from build123d import *

# Parameters (mm, degrees)
BOSS_EXTRUDE1_DEPTH = 3


with BuildPart() as part:
    # Sketch1 → Boss-Extrude1 (new body)
    with BuildSketch(Plane.XY):
        with BuildLine():
            Line((-5, -4), (-5, 4))
            ThreePointArc((-5, 4), (0, 9), (5, 4))
            Line((5, 4), (5, -4))
            ThreePointArc((5, -4), (0, -9), (-5, -4))
        make_face()
        Polygon((1.616580754, 1.2), (3.233161507, 4), (1.616580754, 6.8), (-1.616580754, 6.8), (-3.233161507, 4), (-1.616580754, 1.2), align=None, mode=Mode.SUBTRACT)
        Polygon((3.233161507, -4), (1.616580754, -1.2), (-1.616580754, -1.2), (-3.233161507, -4), (-1.616580754, -6.8), (1.616580754, -6.8), align=None, mode=Mode.SUBTRACT)
    extrude(amount=BOSS_EXTRUDE1_DEPTH)


solid = part.part
Design review of the part built by this model. Coordinates are the model's own, in mm. A direction names the side the tool comes from. Round coordinates to 2 decimals unless told otherwise and drop trailing zeros. Write each loop counter-clockwise with the first axis right and the second up, starting at its lowest first coordinate (ties: lowest second). Pieces come first, ordered by that corner, then holes. Notation, with made-up numbers: (39, 80.25) -> (62, 80.25) arc R25 ccw to (62, 113.25) -> close; hole circle Ø5 at (-30, 20). An arc over 180 degrees is marked (long way). One line per question, with ' | ' between items.
(1) Take a section at C-C, the plane y = 2.75. State the section outline as (x, z) points.
Result sheet:
outline: (-5, 0) -> (-2.51, 0) -> (-2.51, 3) -> (-5, 3) -> close; (2.51, 0) -> (5, 0) -> (5, 3) -> (2.51, 3) -> close
(2) Take a section at D-D, the plane y = -7. State the section outline as (x, z) points, and give its area (3 significant figures).
Result sheet:
outline: (-4, 0) -> (4, 0) -> (4, 3) -> (-4, 3) -> close | area: 24.0 mm2
(3) Wall thickness on line 1 (Y direction, x = 2.25, z = 0.6); line 2 (Y direction, x = 0, z = 1); line 3 (X direction, y = -5.5, z = 1.15): over which ranges is each line inside the solid? List them lowest first. Write a range as [from, to].
Result sheet:
line 1: [-8.47, -5.7], [-2.3, 2.3], [5.7, 8.47] | line 2: [-9, -6.8], [-1.2, 1.2], [6.8, 9] | line 3: [-4.77, -2.37], [2.37, 4.77]
(4) Draft analysis for pull direction Y (two halves, no side actions). For faces 3 (the flat face through (-2.436, 2.62, 1.479)), 4 (the cylindrical face through (0, -9, 1)), 5 (the flat face through (-5, 0, 1)), state which applies: released by +Y, released by -Y, zero draft, split by the parting line, or undercut.
Result sheet:
face 3: undercut | face 4: released by -Y | face 5: zero draft
(5) Take a section at B-B, the plane z = 1.2. State the section outline as (x, y) points, and give its area (3 significant figures).
Result sheet:
outline: (-5, -4) arc R5 ccw to (5, -4) -> (5, 4) arc R5 ccw to (-5, 4) -> close; hole (-3.23, -4) -> (-1.62, -6.8) -> (1.62, -6.8) -> (3.23, -4) -> (1.62, -1.2) -> (-1.62, -1.2) -> close; hole (-3.23, 4) -> (-1.62, 1.2) -> (1.62, 1.2) -> (3.23, 4) -> (1.62, 6.8) -> (-1.62, 6.8) -> close | area: 104 mm2
(6) Insertion check: P1, Ø1.5, axis at y = 5, z = 2.5, coming from the -X side. The pin has a flat end and moves straight along its axis. Give the tip position at first contact, or say it passes through.
Result sheet:
P1: x = -4.99
(7) Machinability: for faces 1 (the flat face through (2.414, -5.42, 1.479)), 2 (the flat face through (0, 0, 3)), which of the approach directions +Z, -Z, +X, -X, +Y, -Y give a long, thin tool a straight path to every point of the face, cutting with its end or side? Answer none if there is none.
Result sheet:
face 1: +Z, -Z | face 2: +Z, +X, -X, +Y, -Y
(8) Take a section at A-A, the plane x = 0. State the section outline as (y, z) points.
Result sheet:
outline: (-9, 0) -> (-6.8, 0) -> (-6.8, 3) -> (-9, 3) -> close; (-1.2, 0) -> (1.2, 0) -> (1.2, 3) -> (-1.2, 3) -> close; (6.8, 0) -> (9, 0) -> (9, 3) -> (6.8, 3) -> close
